```python
from build123d import *

# Parameters (mm, degrees)
EXTRUDE_1_DEPTH     = 16
CHAMFER_1_SIZE      = 5
SHELL_1_T           = -2.5
CUT_EXTRUDE_1_DEPTH = 1.2
SKETCH_3_R          = 5
EXTRUDE_2_DEPTH     = 12.5
CUT_EXTRUDE_2_DEPTH = 2.4
SKETCH_5_R          = 1.6
CUT_EXTRUDE_3_DEPTH = 6
CHAMFER_2_SIZE      = 1


with BuildPart() as part:
    # 草图1 → 凸台-拉伸1 (new body)
    with BuildSketch(Plane.XY):
        with BuildLine():
            ThreePointArc((-14.25, 0), (-20.840097423, 15.909902577), (-36.75, 22.5))
            Line((-36.75, 22.5), (-36.75, -22.5))
            ThreePointArc((-36.75, -22.5), (-20.840097423, -15.909902577), (-14.25, 0))
        make_face()
        with BuildLine():
            Line((-36.75, -22.5), (-36.75, 22.5))
            ThreePointArc((-36.75, 22.5), (-59.25, 0), (-36.75, -22.5))
        make_face()
        with BuildLine():
            Line((36.75, 22.5), (-36.75, 22.5))
            ThreePointArc((-36.75, 22.5), (-20.840097423, 15.909902577), (-14.25, 0))
            ThreePointArc((-14.25, 0), (-20.840097423, -15.909902577), (-36.75, -22.5))
            Line((-36.75, -22.5), (36.75, -22.5))
            Line((36.75, -22.5), (36.75, 22.5))
        make_face()
    extrude(amount=EXTRUDE_1_DEPTH)

    # 倒角1
    chamfer_1_edges = [part.edges().sort_by_distance(p)[0] for p in [
        (0, -22.5, 16),
        (36.75, 0, 16),
        (0, 22.5, 16),
        (-59.25, 0, 16),
    ]]
    chamfer(chamfer_1_edges, length=CHAMFER_1_SIZE)

    # 抽壳1
    shell_1_openings = [part.faces().sort_by_distance(p)[0] for p in [
        (-8.974037689, 0, 0),
    ]]
    offset(amount=SHELL_1_T, openings=shell_1_openings, kind=Kind.INTERSECTION)

    # 草图2 → 切除-拉伸1 (cut)
    with BuildSketch(Plane(origin=(0, 0, 0), x_dir=(-1, 0, 0), z_dir=(0, 0, -1))):
        with BuildLine():
            Line((36.75, 21.2), (-35.45, 21.2))
            Line((-35.45, 21.2), (-35.45, -21.2))
            Line((-35.45, -21.2), (36.75, -21.2))
            ThreePointArc((36.75, -21.2), (57.95, 0), (36.75, 21.2))
        make_face()
        with BuildLine():
            Line((36.75, -20), (-34.25, -20))
            Line((-34.25, -20), (-34.25, 20))
            Line((-34.25, 20), (36.75, 20))
            ThreePointArc((36.75, 20), (56.75, 0), (36.75, -20))
        make_face(mode=Mode.SUBTRACT)
    extrude(amount=-CUT_EXTRUDE_1_DEPTH, mode=Mode.SUBTRACT)

    # 草图3 → 凸台-拉伸2 (add)
    with BuildSketch(Plane(origin=(0, 0, 13.5), x_dir=(-1, 0, 0), z_dir=(0, 0, -1))):
        with Locations(Location((11.25, 0, 0), (0, 0, 180))):
            Circle(SKETCH_3_R)
    extrude(amount=EXTRUDE_2_DEPTH)

    # 草图4 → 切除-拉伸2 (cut)
    with BuildSketch(Plane(origin=(0, 0, 1), x_dir=(-1, 0, 0), z_dir=(0, 0, -1))):
        Polygon((9.66228676, -2.75), (12.83771324, -2.75), (14.425426481, 0), (12.83771324, 2.75), (9.66228676, 2.75), (8.074573519, 0), align=None)
    extrude(amount=-CUT_EXTRUDE_2_DEPTH, mode=Mode.SUBTRACT)

    # 草图5 → 切除-拉伸3 (cut)
    with BuildSketch(Plane(origin=(0, 0, 3.4), x_dir=(-1, 0, 0), z_dir=(0, 0, -1))):
        with Locations((11.25, 0)):
            Circle(SKETCH_5_R)
    extrude(amount=-CUT_EXTRUDE_3_DEPTH, mode=Mode.SUBTRACT)

    # 倒角2
    chamfer_2_edges = [part.edges().sort_by_distance(p)[0] for p in [
        (36.75, -22.5, 5.5),
        (36.75, 22.5, 5.5),
    ]]
    chamfer(chamfer_2_edges, length=CHAMFER_2_SIZE)


solid = part.part
```
The listing builds one solid part. Answer for the finished solid, in the listing's coordinates (mm). A direction names the side the tool comes from. Coordinates: 2 decimals unless noted, no trailing zeros. Loops run counter-clockwise (first coordinate to the right, second up) from the corner with the lowest first, then second, coordinate; pieces in that order, holes last. Notation, with made-up numbers: (-29, 36) -> (16, 36) arc R32 cw to (16, 66) -> close; hole circle Ø3 at (-17, 54). An arc over 180 degrees is marked (long way). Use one line per item in the form item = value. Start each with the question number.
Item 1: The part is cut by section A-A on x = -11.25. Determine the outline of the cut face in (y, z), then the cut area to 3 significant figures.
Item 2: The mould has two halves that part along X. Classify faces 3 (the face through (36.75, 0, 5)), 4 (the face through (-2, -20, 6)), 5 (the face through (0.3, 20, 13.5)): released by +X, released by -X, zero draft, split by the parting line, or undercut.
Item 3: The part is cut by section C-C on x = 12. Determine the outline of the cut face in (y, z), then the cut area to 3 significant figures.
Item 4: A tool of negligible diameter and unlimited length cuts with its end or side. For faces 1 (the face through (-0.8, -20, 13.5)), 2 (the face through (-11, 0, 9.4)), from which of +Z, -Z, +X, -X, +Y, -Y can it reach the whole face along a straight path? Write none if from no direction.
Item 5: The part is cut by section B-B on z = 15. Determine the outline of the cut face in (x, y), then the cut area to 3 significant figures.
Item 6: Flat-ended cylindrical pins translate along their axes: pin 1 Ø21 at (x, y) = (-30.5, 10) entering from -Z; pin 2 Ø1.3 at (y, z) = (-4.5, 1) entering from -X; pin 3 Ø11 at (x, y) = (-12, 1.5) entering from -Z. Find the tip coordinate at first contact, or state that the pin passes through.
Item 7: Consider L1, parallel to Y at x = -11.25, z = 7.05; L2, parallel to Y at x = -5.5, z = 8; L3, parallel to Z at x = -4.5, y = 12.5. Determine where each line is inside the solid, lowest interval first. Write a range as [from, to].
Answer key:
q1.outline = (-22.5, 0) -> (-21.2, 0) -> (-21.2, 1.2) -> (-20, 1.2) -> (-20, 9.96) -> (-16.46, 13.5) -> (-5, 13.5) -> (-5, 1) -> (-2.75, 1) -> (-2.75, 3.4) -> (-1.6, 3.4) -> (-1.6, 9.4) -> (1.6, 9.4) -> (1.6, 3.4) -> (2.75, 3.4) -> (2.75, 1) -> (5, 1) -> (5, 13.5) -> (16.46, 13.5) -> (20, 9.96) -> (20, 1.2) -> (21.2, 1.2) -> (21.2, 0) -> (22.5, 0) -> (22.5, 11) -> (17.5, 16) -> (-17.5, 16) -> (-22.5, 11) -> close
q1.area = 257 mm2
q2.face_3 = released by +X
q2.face_4 = undercut
q2.face_5 = zero draft
q3.outline = (-22.5, 0) -> (-21.2, 0) -> (-21.2, 1.2) -> (-20, 1.2) -> (-20, 9.96) -> (-16.46, 13.5) -> (16.46, 13.5) -> (20, 9.96) -> (20, 1.2) -> (21.2, 1.2) -> (21.2, 0) -> (22.5, 0) -> (22.5, 11) -> (17.5, 16) -> (-17.5, 16) -> (-22.5, 11) -> close
q3.area = 165 mm2
q4.face_1 = +Z, +X, -X, -Y
q4.face_2 = -Z
q5.outline = (-36.75, -18.5) -> (32.75, -18.5) -> (32.75, 18.5) -> (-36.75, 18.5) arc R18.5 ccw to start
q5.area = 3,110 mm2
q6.pin_1 = 1.2
q6.pin_2 = -58.92
q6.pin_3 = 1
q7.L1 = [-22.5, -20], [-5, -1.6], [1.6, 5], [20, 22.5]
q7.L2 = [-22.5, -20], [20, 22.5]
q7.L3 = [13.5, 16]
